Verification items for the finished model (mm, model axes). Round coordinates to 2 decimals unless told otherwise and drop trailing zeros. Write each loop counter-clockwise with the first axis right and the second up, starting at its lowest first coordinate (ties: lowest second). Pieces come first, ordered by that corner, then holes. Notation, with made-up numbers: (58, 30) - (114, 30) arc R16 cw to (114, 55) - close; hole circle Ø7 at (31.5, 69). An arc over 180 degrees is marked (long way). Answer as a JSON object with one key per item and string values.
```python
from build123d import *

# Parameters (mm, degrees)
SKETCH1_R           = 1.85
SKETCH1_R_2         = 50
BOSS_EXTRUDE1_DEPTH = 6.35


with BuildPart() as part:
    # Sketch1 → Boss-Extrude1 (new body)
    with BuildSketch(Plane(origin=(0, 0, 0), x_dir=(1, 0, 0), z_dir=(0, 1, 0))):
        with BuildLine():
            Line((77.567379868, -113.774878941), (81.895896581, -121.29702529))
            Line((81.895896581, -121.29702529), (81.904324829, -121.31160095))
            ThreePointArc((81.904324829, -121.31160095), (83.049348254, -124.303633996), (83.189448927, -127.504213973))
            ThreePointArc((83.189448927, -127.504213973), (83.064062558, -128.818339264), (82.996609195, -130.136708357))
            ThreePointArc((82.996609195, -130.136708357), (79, -136.832013798), (71.203390805, -136.94552617))
            ThreePointArc((71.203390805, -136.94552617), (70.027922997, -136.344757949), (68.827163927, -135.796283084))
            ThreePointArc((68.827163927, -135.796283084), (66.125430696, -134.074662353), (64.106765781, -131.587026457))
            Line((64.106765781, -131.587026457), (64.101233791, -131.577414018))
            Line((64.101233791, -131.577414018), (59.601233791, -123.783185384))
            ThreePointArc((59.601233791, -123.783185384), (55.026304797, -121.940521916), (52.14020721, -125.939999968))
            ThreePointArc((52.14020721, -125.939999968), (50.889960833, -131.187577731), (47.09575677, -135.022183828))
            ThreePointArc((47.09575677, -135.022183828), (44.098818948, -135.114328678), (41.588023883, -133.475415889))
            ThreePointArc((41.588023883, -133.475415889), (36.408246185, -129.437759004), (30, -128))
            Line((30, -128), (-30, -128))
            ThreePointArc((-30, -128), (-36.408246185, -129.437759004), (-41.588023883, -133.475415889))
            ThreePointArc((-41.588023883, -133.475415889), (-44.098818948, -135.114328677), (-47.09575677, -135.022183828))
            ThreePointArc((-47.09575677, -135.022183828), (-59.351969188, -133.446982526), (-71.203390805, -136.94552617))
            ThreePointArc((-71.203390805, -136.94552617), (-79, -136.832013798), (-82.996609195, -130.136708357))
            ThreePointArc((-82.996609195, -130.136708357), (-85.892492332, -118.123804344), (-93.384762884, -108.297213687))
            ThreePointArc((-93.384762884, -108.297213687), (-94.963031576, -105.747861824), (-94.799088999, -102.753993121))
            ThreePointArc((-94.799088999, -102.753993121), (-93.892264414, -96.249345606), (-95.851251684, -89.980762113))
            Line((-95.851251684, -89.980762113), (-125.851251684, -38.019237886))
            ThreePointArc((-125.851251684, -38.019237886), (-130.300510599, -33.188413398), (-136.387112883, -30.721422769))
            ThreePointArc((-136.387112883, -30.721422769), (-139.061850524, -29.366466853), (-140.480519654, -26.724970141))
            ThreePointArc((-140.480519654, -26.724970141), (-145.24446152, -15.323178182), (-154.2, -6.808817812))
            ThreePointArc((-154.2, -6.808817812), (-158, 0), (-154.2, 6.808817812))
            ThreePointArc((-154.2, 6.808817812), (-145.24446152, 15.323178182), (-140.480519654, 26.72497014))
            ThreePointArc((-140.480519654, 26.72497014), (-139.061850524, 29.366466853), (-136.387112883, 30.721422769))
            ThreePointArc((-136.387112883, 30.721422769), (-130.300510599, 33.188413398), (-125.851251684, 38.019237887))
            Line((-125.851251684, 38.019237887), (-95.851251684, 89.980762114))
            ThreePointArc((-95.851251684, 89.980762114), (-93.892264414, 96.249345606), (-94.799088999, 102.753993121))
            ThreePointArc((-94.799088999, 102.753993121), (-94.963031576, 105.747861824), (-93.384762884, 108.297213687))
            ThreePointArc((-93.384762884, 108.297213687), (-85.892492332, 118.123804344), (-82.996609195, 130.136708357))
            ThreePointArc((-82.996609195, 130.136708357), (-79, 136.832013798), (-71.203390805, 136.94552617))
            ThreePointArc((-71.203390805, 136.94552617), (-59.351969188, 133.446982526), (-47.09575677, 135.022183827))
            ThreePointArc((-47.09575677, 135.022183827), (-44.098818948, 135.114328677), (-41.588023883, 133.475415889))
            ThreePointArc((-41.588023883, 133.475415889), (-36.408246185, 129.437759004), (-30, 128))
            Line((-30, 128), (30, 128))
            ThreePointArc((30, 128), (36.408246185, 129.437759004), (41.588023883, 133.475415889))
            ThreePointArc((41.588023883, 133.475415889), (44.098818948, 135.114328677), (47.09575677, 135.022183827))
            ThreePointArc((47.09575677, 135.022183827), (59.351969188, 133.446982526), (71.203390805, 136.94552617))
            ThreePointArc((71.203390805, 136.94552617), (79, 136.832013798), (82.996609195, 130.136708357))
            ThreePointArc((82.996609195, 130.136708357), (85.892492332, 118.123804344), (93.384762884, 108.297213687))
            ThreePointArc((93.384762884, 108.297213687), (94.963031576, 105.747861824), (94.799088999, 102.753993121))
            ThreePointArc((94.799088999, 102.753993121), (93.892264414, 96.249345606), (95.851251684, 89.980762113))
            Line((95.851251684, 89.980762113), (125.851251684, 38.019237886))
            ThreePointArc((125.851251684, 38.019237886), (130.300510599, 33.188413398), (136.387112882, 30.721422769))
            ThreePointArc((136.387112882, 30.721422769), (139.061850524, 29.366466853), (140.480519654, 26.72497014))
            ThreePointArc((140.480519654, 26.72497014), (145.24446152, 15.323178182), (154.2, 6.808817812))
            ThreePointArc((154.2, 6.808817812), (158, 0), (154.2, -6.808817812))
            ThreePointArc((154.2, -6.808817812), (145.24446152, -15.323178182), (140.480519654, -26.72497014))
            ThreePointArc((140.480519654, -26.72497014), (139.061850524, -29.366466853), (136.387112882, -30.721422769))
            ThreePointArc((136.387112882, -30.721422769), (130.300510599, -33.188413399), (125.851251684, -38.019237887))
            Line((125.851251684, -38.019237887), (95.851251684, -89.980762114))
            ThreePointArc((95.851251684, -89.980762114), (93.892264414, -96.249345606), (94.799088999, -102.753993121))
            ThreePointArc((94.799088999, -102.753993121), (94.963031576, -105.747861824), (93.384762884, -108.297213687))
            ThreePointArc((93.384762884, -108.297213687), (88.166794559, -109.665787745), (82.997135719, -108.124743986))
            ThreePointArc((82.997135719, -108.124743986), (77.978753703, -108.736153752), (77.567379868, -113.774878941))
        make_face()
        with Locations((-75, -129.903810568)):
            Circle(SKETCH1_R, mode=Mode.SUBTRACT)
        with Locations((75, -129.903810568)):
            Circle(SKETCH1_R, mode=Mode.SUBTRACT)
        with Locations((150, 0)):
            Circle(SKETCH1_R, mode=Mode.SUBTRACT)
        with Locations((75, 129.903810568)):
            Circle(SKETCH1_R, mode=Mode.SUBTRACT)
        with Locations((-75, 129.903810568)):
            Circle(SKETCH1_R, mode=Mode.SUBTRACT)
        with Locations((-150, 0)):
            Circle(SKETCH1_R, mode=Mode.SUBTRACT)
        Circle(SKETCH1_R_2, mode=Mode.SUBTRACT)
    extrude(amount=BOSS_EXTRUDE1_DEPTH)


solid = part.part
```
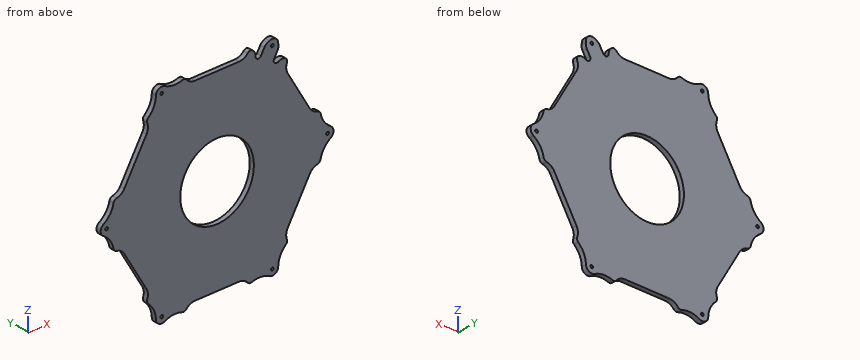
Q1. Section check D-D, the plane x = 108. Record the cut outline in (y, z), then the cut area to 3 significant figures.
Geometry check:
{"outline": "(0, -68.94) - (6.35, -68.94) - (6.35, 68.94) - (0, 68.94) - close", "area": "876 mm2"}
Q2. Section check C-C, the plane z = -70. Record the cut outline in (x, y), then the cut area to 3 significant figures.
Geometry check:
{"outline": "(-107.39, 0) - (107.39, 0) - (107.39, 6.35) - (-107.39, 6.35) - close", "area": "1,360 mm2"}
Q3. Section check A-A, the plane x = 1. Record the cut outline in (y, z), then the cut area to 3 significant figures.
Geometry check:
{"outline": "(0, -128) - (6.35, -128) - (6.35, -49.99) - (0, -49.99) - close; (0, 49.99) - (6.35, 49.99) - (6.35, 128) - (0, 128) - close", "area": "991 mm2"}
Q4. Section check B-B, the plane y = 1.75. State how many separate pieces and enclosed holes the cut face has, then the cut area to 3 significant figures.
Geometry check:
{"separate pieces": "1", "enclosed holes": "7", "area": "51,700 mm2"}
Q5. Gauge pin test, flat ends, axial feed: P1, Ø3, axis at x = -123.5, y = 3, coming from the -Z side; P2, Ø5, axis at x = 75, z = 129.9, coming from the -Y side; P3, Ø3.5, axis at x = -75, z = -129.9, coming from the -Y side; P4, Ø1.9, axis at x = 9, y = 3.5, coming from the -Z side. Record the tip position at first contact, or that the pin passes through.
Geometry check:
{"P1": "stops at z = -44.69", "P2": "stops at y = 0", "P3": "passes through", "P4": "stops at z = -128"}
Q6. Material ranges on line 1 along Z through (x, y) = (75, 1.5); line 2 along Z through (x, y) = (0, 2); line 3 along X through (y, z) = (2, -19), recorded low to high. Write a range as [from, to].
Geometry check:
{"line 1": "z = [-137.9, -131.75], [-128.05, 128.05], [131.75, 137.9]", "line 2": "z = [-128, -50], [50, 128]", "line 3": "x = [-143.08, -46.25], [46.25, 143.08]"}
